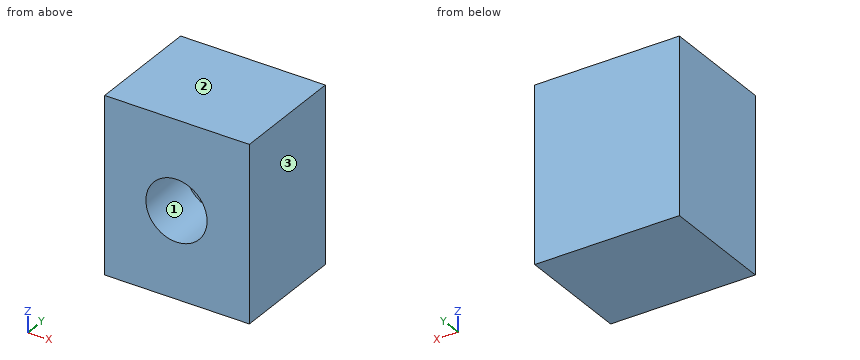
from build123d import *

# Parameters (mm, degrees)
F0_W      = 60.16257
F0_H      = 62.742576
F1_DEPTH  = 48
F1_FACE_W = 60.16257
F1_FACE_H = 48
F2_DEPTH  = 10
F4_R      = 12.38494
F5_DEPTH  = 30
F3_R      = 12.720557
F6_DEPTH  = 25


with BuildPart() as f1:
    # F0 (on Front) → F1 (new body)
    with BuildSketch(Plane.XZ):
        with Locations((30.081285, 31.371288)):
            Rectangle(F0_W, F0_H)
    extrude(amount=F1_DEPTH)

    # F1_face (on face) → F2 (join)
    with BuildSketch(Plane(origin=(30.081285, -24, 62.742576), x_dir=(1, 0, 0), z_dir=(0, 0, 1))):
        Rectangle(F1_FACE_W, F1_FACE_H)
    extrude(amount=F2_DEPTH)

    # F4 (on face) → F5 (join)
    with BuildSketch(Plane.XZ.offset(48)):
        with Locations((30.478884, 35.89391)):
            Circle(F4_R)
    extrude(amount=-F5_DEPTH)

    # F3 (on face) → F6 (cut)
    with BuildSketch(Plane.XZ.offset(48)):
        with Locations((29.86002, 35.89391)):
            Circle(F3_R)
    extrude(amount=-F6_DEPTH, mode=Mode.SUBTRACT)


solid = f1.part
The model under review builds one solid part; all positions refer to its coordinate system, in mm. Face numbers are marked on the shaded views. Round coordinates to 2 decimals unless told otherwise and drop trailing zeros. Loops run counter-clockwise (first coordinate to the right, second up) from the corner with the lowest first, then second, coordinate; pieces in that order, holes last. Notation, with made-up numbers: (77.25, 31.5) -> (106.25, 31.5) arc R24 cw to (106.25, 47.5) -> close; hole circle Ø2 at (-32.5, 80.25). An arc over 180 degrees is marked (long way). Return JSON: item names as keys, results as strings.
(1) For line 1 (Y direction, x = 30.5, z = 33); line 2 (X direction, y = -32, z = 32); line 3 (X direction, y = -45, z = 25), list the stretches that pass through material, from the lowest coordinate up.
Solved:
{"line 1": "-23 to 0", "line 2": "0 to 17.75, 41.97 to 60.16", "line 3": "0 to 23.29, 36.43 to 60.16"}
(2) The part is to be moulded in two halves that separate along X. For the marked faces 1, 2 and 3, say which applies: released by +X, released by -X, zero draft, split by the parting line, or undercut.
Solved:
{"face 1": "undercut", "face 2": "zero draft", "face 3": "released by +X"}
(3) Add section A-A on z = 28.5. Write out the cut boundary in (x, y).
Solved:
{"outline": "(0, -48) -> (19.51, -48) -> (19.51, -23) -> (40.21, -23) -> (40.21, -48) -> (60.16, -48) -> (60.16, 0) -> (0, 0) -> close"}
(4) Add section C-C on y = -29.5. Write out the cut boundary in (x, z), plus the area to 3 significant figures.
Solved:
{"outline": "(0, 0) -> (60.16, 0) -> (60.16, 72.74) -> (0, 72.74) -> close; hole circle Ø25.44 at (29.86, 35.89)", "area": "3,870 mm2"}
(5) For pin 1 (7.5 mm diameter, centred on x = 27.5, z = 38.5, fed in from -Y), flat-tipped, find the tip position at first contact; note if it passes through.
Solved:
{"pin 1": "y = -23"}
(6) Add section B-B on x = 19. Write out the cut boundary in (y, z).
Solved:
{"outline": "(-48, 0) -> (0, 0) -> (0, 72.74) -> (-48, 72.74) -> (-48, 42.52) -> (-23, 42.52) -> (-23, 29.27) -> (-48, 29.27) -> close"}
